Part model, mm, in its own coordinate system. A direction names the side the tool comes from. Give positions to 0.01 mm unless a question says otherwise; leave off trailing zeros. Write each loop counter-clockwise with the first axis right and the second up, starting at its lowest first coordinate (ties: lowest second). Pieces come first, ordered by that corner, then holes. Notation, with made-up numbers: M -26.5,-9 L 22.5,-9 A30 ccw 22.5,27 Z; hole C 61,-19 d9. An arc over 180 degrees is marked long. Answer as CSV lines item,"result". Start each with the question number.
1) Wall check: line 1 along Y through (x, z) = (0.65, 9.5); line 2 along Z through (x, y) = (2.7, -6.5); line 3 along Y through (x, z) = (2.45, -15). Give the ranges that are in metal, low to high. Write a range as from..to.
2) Tool access for faces 4 (the flat face through (1.479, -2.788, 9.718)), 5 (the flat face through (1, -4.389, -10)), 6 (the flat face through (1, -18.009, -10)): list every direction of +Z, -Z, +X, -X, +Y, -Y with a clear straight run to the whole face (end or side of a thin tool).
3) Mould opens along Y. For faces 1 (the cylindrical face through (1.521, -6.166, -19.337)), 2 (the flat face through (1, -11, -22.086)), 3 (the flat face through (1.48, -19.56, 5.41)) say: pulls with the +Y half, pulls with the -Y half, needs draft (parallel to the pull), parting line crosses it, or undercut.
4) Slice it at C-C, the plane y = -12.5. Give the cut face in (x, z), plus the area to 3 significant figures.
5) Slice it at B-B, the plane x = 1.25. Give the cut face in (y, z).
6) Slice it at D-D, the plane y = -3.75. Give the cut face in (x, z).
7) Pin check, flat tips, straight feed: pin 1 Ø1.5 at (x, z) = (1, 6) entering from +Y; pin 2 Ø1 at (x, z) = (2, 4) entering from +Y; pin 3 Ø1.5 at (x, z) = (1.5, -14.5) entering from +Y. Stop position of each tip, or through.
8) Slice it at A-A, the plane z = 11.5. Give the cut face in (x, y), plus the area to 3 significant figures.
```python
from build123d import *

# Parameters (mm, degrees)
BOSS_EXTRUDE1_DEPTH = 3
FILLET1_R           = 0.75
SKETCH3_R           = 0.75
CUT_EXTRUDE1_DEPTH  = 4


with BuildPart() as part:
    # Sketch2 → Boss-Extrude1 (new body)
    with BuildSketch(Plane(origin=(0, 0, 0), x_dir=(0, 0, -1), z_dir=(1, 0, 0))):
        Polygon((-20.913575794, -4.388518255), (-8.919601915, -4.388518255), (-10.913575794, -0.388518255), (-1.919601915, -4.388518255), (22.086424206, -4.388518255), (22.086424206, -18.00920791), (-1.919601915, -18.00920791), (-10.913575794, -22.00920791), (-8.919601915, -18.00920791), (-20.913575794, -18.00920791), (-20.913575794, -13.698863083), (15.086424206, -13.698863083), (15.086424206, -8.698863083), (-20.913575794, -8.698863083), align=None)
    extrude(amount=BOSS_EXTRUDE1_DEPTH)

    # Fillet1
    fillet1_edges = [part.edges().sort_by_distance(p)[0] for p in [
        (1.5, -4.388518255, 8.919601915),
        (1.5, -0.388518255, 10.913575794),
        (1.5, -22.00920791, 10.913575794),
        (1.5, -18.00920791, 8.919601915),
    ]]
    fillet(fillet1_edges, radius=FILLET1_R)

    # Sketch3 → Cut-Extrude1 (cut, through all)
    with BuildSketch(Plane(origin=(3, 0, 0), x_dir=(0, 0, -1), z_dir=(1, 0, 0))):
        with Locations((20.086424206, -6.198863083)):
            Circle(SKETCH3_R)
        with Locations((20.086424206, -16.198863083)):
            Circle(SKETCH3_R)
        with Locations((20.086424206, -11.198863083)):
            Circle(SKETCH3_R)
        with Locations((12.586424206, -6.198863083)):
            Circle(SKETCH3_R)
        with Locations((12.586424206, -16.198863083)):
            Circle(SKETCH3_R)
    extrude(amount=-CUT_EXTRUDE1_DEPTH, mode=Mode.SUBTRACT)


solid = part.part
```
Found:
1,line 1,"-21.2..-19.17, -18.35..-13.7, -8.7..-4.04, -3.22..-1.2"
1,line 2,"-22.09..-20.77, -19.4..-13.27, -11.9..20.91"
1,line 3,"-18.01..-13.7, -8.7..-4.39"
2,face 4,"+Z, +X, -X"
2,face 5,"-Z, +X, -X, +Y"
2,face 6,"-Z, +X, -X, -Y"
3,face 1,"undercut"
3,face 2,"needs draft"
3,face 3,"pulls with the -Y half"
4,outline,"M 0,-22.09 L 3,-22.09 L 3,-15.09 L 0,-15.09 Z"
4,area,"21.0 mm²"
5,outline,"M -21.16,9.01 L -18.01,1.92 L -18.01,-22.09 L -4.39,-22.09 L -4.39,1.92 L -1.24,9.01 A0.75 ccw -2.26,9.98 L -3.3,9.46 A0.75 cw -4.39,10.13 L -4.39,20.91 L -8.7,20.91 L -8.7,-15.09 L -13.7,-15.09 L -13.7,20.91 L -18.01,20.91 L -18.01,10.13 A0.75 cw -19.09,9.46 L -20.14,9.98 A0.75 ccw Z; hole C -16.2,-20.09 d1.5; hole C -16.2,-12.59 d1.5; hole C -11.2,-20.09 d1.5; hole C -6.2,-20.09 d1.5; hole C -6.2,-12.59 d1.5"
6,outline,"M 0,3.36 L 3,3.36 L 3,9.39 L 0,9.39 Z"
7,pin 1,"y = -2.24"
7,pin 2,"y = -3.24"
7,pin 3,"y = -4.39"
8,outline,"M 0,-18.01 L 3,-18.01 L 3,-13.7 L 0,-13.7 Z; M 0,-8.7 L 3,-8.7 L 3,-4.39 L 0,-4.39 Z"
8,area,"25.9 mm²"
